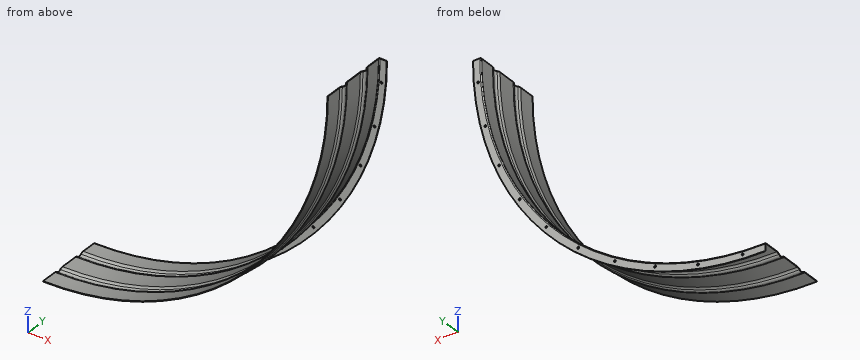
from build123d import *

# Parameters (mm, degrees)
REVOLVE1_ANGLE     = 90
SKETCH2_R          = 7
CUT_EXTRUDE1_DEPTH = 2719.294935026
CIRPATTERN1_COUNT  = 10
CIRPATTERN1_ANGLE  = 81


with BuildPart() as part:
    # Sketch1 → Revolve1 (revolve)
    with BuildSketch(Plane(origin=(0, 0, 0), x_dir=(0, 0, -1), z_dir=(1, 0, 0))):
        with BuildLine():
            ThreePointArc((1668.18678357, 678.502698393), (1663.349291107, 670.794245847), (1661.659054885, 661.851948853))
            Line((1661.659054885, 661.851948853), (1661.659054885, 548.005358054))
            Line((1661.659054885, 548.005358054), (1658.659054885, 548.005358054))
            Line((1658.659054885, 548.005358054), (1658.659054885, 661.851948852))
            ThreePointArc((1658.659054885, 661.851948852), (1660.556258803, 671.889220983), (1665.986097271, 680.541565679))
            ThreePointArc((1665.986097271, 680.541565679), (1672.827265195, 697.483265753), (1666.680039152, 714.688915753))
            ThreePointArc((1666.680039152, 714.688915753), (1660.728201813, 724.848073855), (1658.659054648, 736.439082916))
            Line((1658.659054648, 736.439082916), (1658.659054648, 861.851948852))
            ThreePointArc((1658.659054648, 861.851948852), (1660.556258566, 871.889220983), (1665.986097033, 880.541565679))
            ThreePointArc((1665.986097033, 880.541565679), (1672.827264958, 897.483265753), (1666.680038915, 914.688915753))
            ThreePointArc((1666.680038915, 914.688915753), (1660.728201582, 924.848073824), (1658.659054411, 936.439082853))
            Line((1658.659054411, 936.439082853), (1658.659054411, 1040.005358054))
            ThreePointArc((1658.659054411, 1040.005358054), (1661.002200161, 1045.662212304), (1666.659054411, 1048.005358054))
            Line((1666.659054411, 1048.005358054), (1713.659054411, 1048.005358054))
            Line((1713.659054411, 1048.005358054), (1713.659054411, 1045.005358054))
            Line((1713.659054411, 1045.005358054), (1666.659054411, 1045.005358054))
            ThreePointArc((1666.659054411, 1045.005358054), (1663.123520505, 1043.54089196), (1661.659054411, 1040.005358054))
            Line((1661.659054411, 1040.005358054), (1661.659054411, 936.439082853))
            ThreePointArc((1661.659054411, 936.439082853), (1663.54290482, 925.886074633), (1668.961741794, 916.636691913))
            ThreePointArc((1668.961741794, 916.636691913), (1675.826645674, 897.422312329), (1668.186783333, 878.502698393))
            ThreePointArc((1668.186783333, 878.502698393), (1663.349290869, 870.794245847), (1661.659054648, 861.851948853))
            Line((1661.659054648, 861.851948853), (1661.659054648, 736.43908291))
            ThreePointArc((1661.659054648, 736.43908291), (1663.542905053, 725.88607466), (1668.961742034, 716.636691911))
            ThreePointArc((1668.961742034, 716.636691911), (1675.826645911, 697.422312328), (1668.18678357, 678.502698393))
        make_face()
    revolve(axis=Axis((0, 1001.495453618, 336.340945352), (0, -1, 0)), revolution_arc=REVOLVE1_ANGLE)

    # Sketch2 → Cut-Extrude1 (cut, symmetric)
    with BuildSketch(Plane(origin=(0, 1048.005358054, 0), x_dir=(1, 0, 0), z_dir=(0, 1, 0))):
        with Locations(Location((158.48737337, 1677.432068789, 0), (0, 0, 90))):
            Circle(SKETCH2_R)
    cut_extrude1 = extrude(amount=CUT_EXTRUDE1_DEPTH, both=True, mode=Mode.SUBTRACT)

    # CirPattern1: Cut-Extrude1 ×10 about axis
    cirpattern1_axis = Axis((0, 0, 336.340945352), (0, -1, 0))
    for i in range(1, CIRPATTERN1_COUNT):
        add(cut_extrude1.rotate(cirpattern1_axis, i * CIRPATTERN1_ANGLE / (CIRPATTERN1_COUNT - 1)), mode=Mode.SUBTRACT)


solid = part.part
For this review, take the finished solid that the model builds, in its own axes (mm). Round coordinates to 2 decimals unless told otherwise and drop trailing zeros. Loops run counter-clockwise (first coordinate to the right, second up) from the corner with the lowest first, then second, coordinate; pieces in that order, holes last. Notation, with made-up numbers: (-19.5, 78.5) - (3.5, 78.5) arc R16 ccw to (3.5, 85.5) - close; hole circle Ø11 at (5, 75). An arc over 180 degrees is marked (long way). Answer as CSV lines item,"result".
(1) Wall thickness on line 1 (X direction, y = 910, z = -20); line 2 (Z direction, x = 986.5, y = 759); line 3 (Z direction, x = 1846, y = 631): over which ranges is each line inside the solid? List them lowest first.
Checked values:
line 1,"x = 1974.3 to 1977.7"
line 2,"z = -1401.13 to -1397.68"
line 3,"z = -428.05 to -420.17"
(2) Consider section A-A on y = 971.5. Give the boundary of the cut face in (x, z).
Checked values:
outline,"(0, -1661.66) arc R1998 ccw to (1998, 336.34) - (1995, 336.34) arc R1995 cw to (0, -1658.66) - close"
(3) Insertion check: P1, Ø22.5, axis at x = 773.02, z = -1529.9, coming from the -Y side; P2, Ø8.5, axis at x = 1866.24, z = -436.68, coming from the +Y side; P3, Ø2, axis at y = 939.5, z = -618.5, coming from the +X side; P4, Ø4, axis at y = 741, z = -568.5, coming from the +X side. Each pin has a flat end and moves straight along its axis. Give the tip position at first contact, or say it passes through.
Checked values:
P1,"stops at y = 684.42"
P2,"passes through"
P3,"stops at x = 1755.62"
P4,"stops at x = 1782.38"
